Geometry: final body of the model. Coordinates: model frame, mm. Give positions to 0.01 mm unless a question says otherwise; leave off trailing zeros. Loops run counter-clockwise (first coordinate to the right, second up) from the corner with the lowest first, then second, coordinate; pieces in that order, holes last.
1. Section A-A, the plane y = 0. Output: boundary loops of the cut face in (x, z).
2. First-contact query: P1, Ø1.8, axis at x = 0, y = 0, coming from the +Z side; P2, Ø3, axis at y = 1, z = 21.5, coming from the -X side; P3, Ø0.9, axis at x = 0.5, y = 0, coming from the -Z side; P4, Ø3, axis at x = 2, z = 11.5, coming from the +Y side. Flat tips, straight axial feed; report the tip coordinate or a pass-through.
3. Material intervals for line 1 along Y through (x, z) = (0, 43.15); line 2 along X through (y, z) = (2.6, 31); line 3 along Y through (x, z) = (-1, 3), sorted ascending.
4. Section C-C, the plane z = 16.5. Output: boundary loops of the cut face in (x, y), then the cut area to 3 significant figures.
5. Section D-D, the plane y = 2.5. Output: boundary loops of the cut face in (x, z), then the cut area to 3 significant figures.
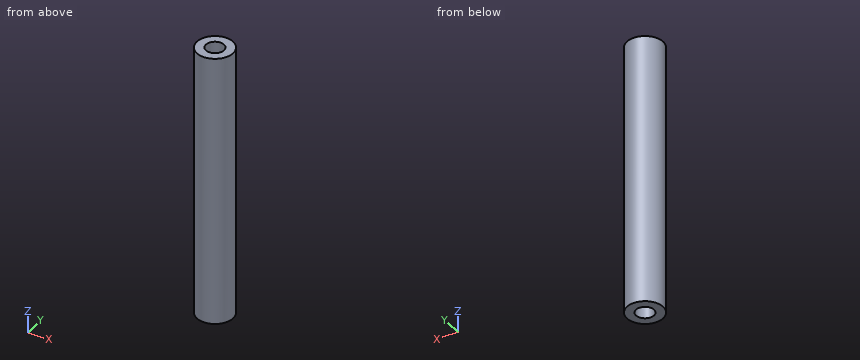
Autodesk Inventor part; units mm, degrees
ref_plane "作業平面1" through (0, 0, 39) normal (0, 0, 1) x (1, 0, 0)
ref_plane "YZ Plane" through (0, 0, 0) normal (1, 0, 0) x (0, 1, 0)
ref_plane "XZ Plane" through (0, 0, 0) normal (0, 1, 0) x (-1, 0, 0)
sketch "スケッチ1" plane through (0, 0, 0) normal (0, 0, 1) x (1, 0, 0)
  circle A0 centre (0, 0) radius 3
  circle A1 centre (0, 0) radius 1.5
  dimension "d0" = 6
  dimension "d1" = 3
extrude "押し出し1" add sketch "スケッチ1" along normal blind 45
ref_plane "作業平面1" through (0, 0, 39) normal (0, 0, 1) x (1, 0, 0)
sketch "スケッチ2" plane through (0, 0, 39) normal (0, 0, 1) x (1, 0, 0)
  point P0 (0, 0)
sketch "スケッチ3" plane through (0, 0, 39) normal (0, 0, 1) x (1, 0, 0)
  circle A0 centre (0, 0) radius 1.5
  circle A1 centre (0, 0) radius 3
extrude "押し出し2" add sketch "スケッチ3" against normal blind 33 contours A0
properties part number "ABSスペーサーm3-45　簡易筒型" material "ABS プラスチック"
Answers below:
1. outline: (-3, 0) - (-1.5, 0) - (-1.5, 6) - (1.5, 6) - (1.5, 0) - (3, 0) - (3, 45) - (1.5, 45) - (1.5, 39) - (-1.5, 39) - (-1.5, 45) - (-3, 45) - close
2. P1: stops at z = 39
2. P2: stops at x = -3
2. P3: stops at z = 6
2. P4: stops at y = 2.96
3. line 1: y = -3 to -1.5, 1.5 to 3
3. line 2: x = -1.5 to 1.5
3. line 3: y = -2.83 to -1.12, 1.12 to 2.83
4. outline: circle Ø6 at (0, 0)
4. area: 28.3 mm2
5. outline: (-1.66, 0) - (1.66, 0) - (1.66, 45) - (-1.66, 45) - close
5. area: 149 mm2
